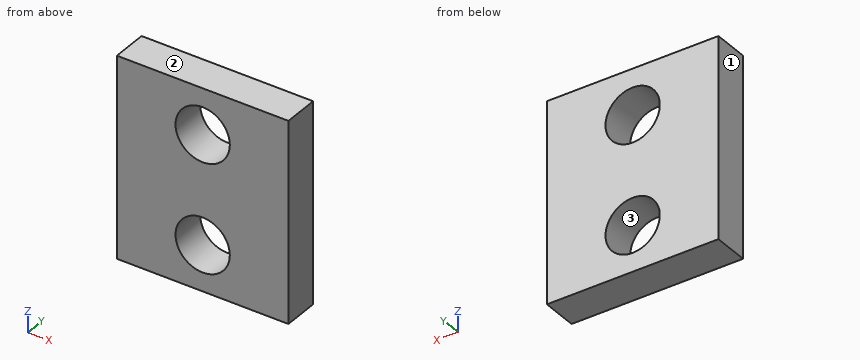
from build123d import *

# Parameters (mm, degrees)
F0_W     = 120
F0_H     = 140
F0_R     = 19
F1_DEPTH = 25
F2_DEPTH = 25


with BuildPart() as f1:
    # F0 (on Front) → F1 (new body)
    with BuildSketch(Plane.XZ):
        Rectangle(F0_W, F0_H)
        with Locations((0, -38)):
            Circle(F0_R, mode=Mode.SUBTRACT)
        with Locations((0, 38)):
            Circle(F0_R, mode=Mode.SUBTRACT)
    extrude(amount=F1_DEPTH)

    # F0 (on Front) → F2 (cut)
    with BuildSketch(Plane.XZ):
        with Locations((0, 38)):
            Circle(F0_R)
    extrude(amount=F2_DEPTH, mode=Mode.SUBTRACT)


solid = f1.part
Can you work these out from the model? Positions are in its coordinate system, mm. Face numbers are marked on the shaded views. Coordinates: 2 decimals unless noted, no trailing zeros. Loops run counter-clockwise (first coordinate to the right, second up) from the corner with the lowest first, then second, coordinate; pieces in that order, holes last. Notation, with made-up numbers: M 38.25,8.25 L 74.25,8.25 A35 cw 74.25,46.25 Z; hole C 12,52.25 d6. An arc over 180 degrees is marked long. Return JSON: item names as keys, results as strings. Group by question number.
Item 1: Imagine slicing it at B-B (x = 0). Please give me the cut outline in (y, z), and give its area (3 significant figures).
Item 2: Imagine slicing it at C-C (y = -2.25). Please give me the cut outline in (x, z), and give its area (3 significant figures).
Item 3: If I drill on L1, parallel to Z at x = -0.5, y = -8.5; L2, parallel to Z at x = 16, y = -2; L3, parallel to X at y = -16.25, z = 37.5, over which ranges is the centre line in solid material (lowest first)? Write a range as from..to.
Item 4: I'm going to push flat-ended pins straight in: pin 1 Ø23 at (x, z) = (0, 38) entering from -Y; pin 2 Ø10 at (x, z) = (-27, 7) entering from +Y. Where does each tip first touch, or does it pass through?
Item 5: Imagine slicing it at D-D (x = -16.5). Please give me the cut outline in (y, z).
Item 6: Thinking about a two-plate mould opening in X: for the marked faces 1, 2 and 3, which applies, released by +X, released by -X, zero draft, split by the parting line, or undercut?
Item 7: Imagine slicing it at A-A (z = 38). Please give me the cut outline in (x, y).
Verdict:
{
 "1": {"outline": "M -25,-70 L 0,-70 L 0,-57 L -25,-57 Z; M -25,-19 L 0,-19 L 0,19 L -25,19 Z; M -25,57 L 0,57 L 0,70 L -25,70 Z", "area": "1,600 mm^2"},
 "2": {"outline": "M -60,-70 L 60,-70 L 60,70 L -60,70 Z; hole C 0,-38 d38; hole C 0,38 d38", "area": "14,500 mm^2"},
 "3": {"L1": "z = -70..-56.99, -19.01..19.01, 56.99..70", "L2": "z = -70..-48.25, -27.75..27.75, 48.25..70", "L3": "x = -60..-18.99, 18.99..60"},
 "4": {"pin 1": "passes through", "pin 2": "stops at y = 0"},
 "5": {"outline": "M -25,-70 L 0,-70 L 0,-47.42 L -25,-47.42 Z; M -25,-28.58 L 0,-28.58 L 0,28.58 L -25,28.58 Z; M -25,47.42 L 0,47.42 L 0,70 L -25,70 Z"},
 "6": {"face 1": "released by -X", "face 2": "zero draft", "face 3": "undercut"},
 "7": {"outline": "M -60,-25 L -19,-25 L -19,0 L -60,0 Z; M 19,-25 L 60,-25 L 60,0 L 19,0 Z"}
}
